```python
from build123d import *

# Parameters (mm, degrees)
F1_DEPTH = 291
F3_SIZE2 = 25
F3_SIZE  = 9.5
F4_SIZE2 = 10.1
F4_SIZE  = 88
F6_R     = 1.75
F7_DEPTH = 3.2


with BuildPart() as f1:
    # F0 (on Front) → F1 (new body, symmetric)
    with BuildSketch(Plane.XZ):
        Polygon((25.4, 12.7), (22.2, 12.7), (22.2, -9.5), (0, -9.5), (0, -12.7), (25.4, -12.7), align=None)
    extrude(amount=F1_DEPTH, both=True)

    # F3
    f3_edges = [f1.edges().sort_by_distance(p)[0] for p in [
        (23.8, 291, 12.7),
    ]]
    f3_side = f1.faces().sort_by_distance((23.8, 291, 12.34079))[0]
    chamfer(f3_edges, length=F3_SIZE, length2=F3_SIZE2, reference=f3_side)

    # F4
    f4_edges = [f1.edges().sort_by_distance(p)[0] for p in [
        (23.8, -291, 12.7),
    ]]
    f4_side = f1.faces().sort_by_distance((23.8, -12.5, 12.7))[0]
    chamfer(f4_edges, length=F4_SIZE, length2=F4_SIZE2, reference=f4_side)

    # F6 (on face) → F7 (cut, through all)
    with BuildSketch(Plane.XY.offset(-9.5)):
        with Locations((12.7, -283.8)):
            Circle(F6_R)
        with Locations((12.7, 283.8)):
            Circle(F6_R)
    extrude(amount=-F7_DEPTH, mode=Mode.SUBTRACT)


solid = f1.part
```
Geometry: final body of the model. Coordinates: model frame, mm. A direction names the side the tool comes from. Give positions to 0.01 mm unless a question says otherwise; leave off trailing zeros. Write each loop counter-clockwise with the first axis right and the second up, starting at its lowest first coordinate (ties: lowest second). Pieces come first, ordered by that corner, then holes.
1. Pin query (flat end, axial travel): P1, Ø1, axis at x = 14, y = -13, coming from the +Z side; P2, Ø5.5, axis at x = 12.7, y = 283.8, coming from the -Z side; P3, Ø11, axis at y = -22, z = 5.5, coming from the -X side; P4, Ø3, axis at x = 12.7, y = -283.8, coming from the +Z side. Return the tip coordinate at first contact, or that it passes through.
2. Section query C-C, the plane x = 5.5. Return loops of the section in (y, z), then the cut area to 3 significant figures.
3. Reachability of faces 1 (the flat face through (23.82, -247.62, 7.58)), 2 (the flat face through (11, -4, -9.5)) from +Z, -Z, +X, -X, +Y, -Y: full face, straight path, thin tool, end or side. Return the list, or none.
4. Section query B-B, the plane y = -193.5. Return loops of the section in (x, z).
5. Line query: probe 1 along Y at (x, z) = (12.7, -11.45); probe 2 along X at (y, z) = (-283.8, -11.2); probe 3 along X at (y, z) = (13, 11.5). Output: solid intervals per line, ascending.
6. Section query A-A, the plane z = -5.5. Return loops of the section in (x, y).
Computed:
1. P1: stops at z = -9.5
1. P2: stops at z = -12.7
1. P3: stops at x = 22.2
1. P4: passes through
2. outline: (-291, -12.7) - (291, -12.7) - (291, -9.5) - (-291, -9.5) - close
2. area: 1,860 mm2
3. face 1: +Z, +X, -X, -Y
3. face 2: +Z, -X, +Y, -Y
4. outline: (0, -12.7) - (25.4, -12.7) - (25.4, 12.7) - (22.2, 12.7) - (22.2, -9.5) - (0, -9.5) - close
5. probe 1: y = -291 to -285.55, -282.05 to 282.05, 285.55 to 291
5. probe 2: x = 0 to 10.95, 14.45 to 25.4
5. probe 3: x = 22.2 to 25.4
6. outline: (22.2, -291) - (25.4, -291) - (25.4, 291) - (22.2, 291) - close
